from build123d import *

# Parameters (mm, degrees)
BOSS_EXTRUDE1_DEPTH = 1
SKETCH2_R           = 0.411394619
SKETCH2_R_2         = 0.305784332
SKETCH2_R_3         = 0.294014574
SKETCH2_R_4         = 0.29238352
SKETCH2_R_5         = 0.265611248
SKETCH2_R_6         = 0.339655263
SKETCH2_R_7         = 0.419941145
SKETCH2_R_8         = 0.432128273
CUT_EXTRUDE1_DEPTH  = 1
SKETCH2_5_R         = 2.453911785
BOSS_EXTRUDE2_DEPTH = 4


with BuildPart() as part:
    # Sketch1 → Boss-Extrude1 (new body)
    with BuildSketch(Plane.XY):
        with BuildLine():
            Line((-6.5, -5), (6.5, -5))
            ThreePointArc((6.5, -5), (7.207106781, -4.707106781), (7.5, -4))
            Line((7.5, -4), (7.5, 4))
            ThreePointArc((7.5, 4), (7.207106781, 4.707106781), (6.5, 5))
            Line((6.5, 5), (-6.5, 5))
            ThreePointArc((-6.5, 5), (-7.207106781, 4.707106781), (-7.5, 4))
            Line((-7.5, 4), (-7.5, -4))
            ThreePointArc((-7.5, -4), (-7.207106781, -4.707106781), (-6.5, -5))
        make_face()
    extrude(amount=BOSS_EXTRUDE1_DEPTH)

    # Sketch2 → Cut-Extrude1 (cut)
    with BuildSketch(Plane.XY.offset(1)):
        with Locations((-6.6069869, -4.252731437)):
            Circle(SKETCH2_R)
        with Locations((-2.739976181, -3.037963672)):
            Circle(SKETCH2_R_2)
        with Locations((-0.911075824, -2.990722704)):
            Circle(SKETCH2_R_3)
        with Locations((0.789599047, -2.990722704)):
            Circle(SKETCH2_R_4)
        with Locations((2.510520048, -2.990722704)):
            Circle(SKETCH2_R_5)
        with Locations((6.667725288, -4.252731437)):
            Circle(SKETCH2_R_6)
        with Locations((6.667725288, 4.061679043)):
            Circle(SKETCH2_R_7)
        with Locations((-6.6069869, 4.061679043)):
            Circle(SKETCH2_R_8)
    extrude(amount=-CUT_EXTRUDE1_DEPTH, mode=Mode.SUBTRACT)

    # Sketch2_5 → Boss-Extrude2 (add)
    with BuildSketch(Plane.XY.offset(1)):
        with Locations(Location((0, 0, 0), (0, 0, 180))):
            Circle(SKETCH2_5_R)
    extrude(amount=BOSS_EXTRUDE2_DEPTH)

    # Sketch6 → Revolve1 (revolve)
    with BuildSketch(Plane(origin=(0, 0, 0), x_dir=(0, 0, -1), z_dir=(1, 0, 0)), mode=Mode.PRIVATE) as revolve1_sk:
        Polygon((-5, 2.453911785), (-8.647016012, 2.453911785), (-8.647016012, 1.874818049), (-7.823508006, 1.280931587), (-7.823508006, 0), (-5, 0), align=None)
    revolve(revolve1_sk.sketch.rotate(Axis((0, 0, 7.823508006), (0, 0, -1)), 270), axis=Axis((0, 0, 7.823508006), (0, 0, -1)))


solid = part.part
Read the model definition and answer for the solid it produces. Units are mm, in the model's axes. A direction names the side the tool comes from. Round coordinates to 2 decimals unless told otherwise and drop trailing zeros. Loops run counter-clockwise (first coordinate to the right, second up) from the corner with the lowest first, then second, coordinate; pieces in that order, holes last. Notation, with made-up numbers: (74.5, 36.5) - (114.5, 36.5) arc R6 cw to (114.5, 42.5) - close; hole circle Ø4 at (-7, 31). An arc over 180 degrees is marked (long way). One line per question, with ' | ' between items. Start each with the question number.
Q1. Section D-D on z = 5 is taken. Give the vertices of the cut face in (x, y), plus the area to 3 significant figures.
Q2. Section B-B on x = 0 is taken. Give the vertices of the cut face in (y, z).
Q3. Find the intervals of material crossed by L1, parallel to Z at x = 2, y = -4; L2, parallel to X at y = 0, z = 2; L3, parallel to X at y = 0.25, z = 6, in increasing order.
Q4. Section A-A on y = 0 is taken. Give the vertices of the cut face in (x, z).
Q5. Section C-C on z = 0.5 is taken. Count the separate pieces of the cut face and the enclosed holes in it, plus the area to 3 significant figures.
Q6. For a pull along Y with two mould halves and no side action, classify faces 3 (the cylindrical face through (6.25, 4.08, 0.51)), 4 (the cylindrical face through (-6.195, 4.191, 0.507)), 5 (the flat face through (-2, 2, 1)), 6 (the flat face through (0.1, 5, 0.5)) as +Y half, -Y half, draft (parallel to the pull), parting line (faces both ways), or undercut.
Q7. Flat-ended cylindrical pins translate along their axes: pin 1 (2 mm diameter, centred on x = -3.5, y = -2, fed in from +Z); pin 2 (0.8 mm diameter, centred on x = -0.5, y = 0, fed in from +Z). Find the tip coordinate at first contact, or state that the pin passes through.
Q8. For faces 1 (the flat face through (-0.1, -5, 0.5)), 2 (the flat face through (0, 0, 7.824)), determine the directions among +Z, -Z, +X, -X, +Y, -Y from which every point of the face is accessible in a straight line to the end or side of a thin tool.
Established:
1) outline: circle Ø4.91 at (0, 0) | area: 18.9 mm²
2) outline: (-5, 0) - (5, 0) - (5, 1) - (2.45, 1) - (2.45, 8.65) - (1.87, 8.65) - (1.28, 7.82) - (-1.28, 7.82) - (-1.87, 8.65) - (-2.45, 8.65) - (-2.45, 1) - (-5, 1) - close
3) L1: 0 to 1 | L2: -2.45 to 2.45 | L3: -2.44 to 2.44
4) outline: (-7.5, 0) - (7.5, 0) - (7.5, 1) - (2.45, 1) - (2.45, 8.65) - (1.87, 8.65) - (1.28, 7.82) - (-1.28, 7.82) - (-1.87, 8.65) - (-2.45, 8.65) - (-2.45, 1) - (-7.5, 1) - close
5) separate pieces: 1 | enclosed holes: 8 | area: 146 mm²
6) face 3: undercut | face 4: undercut | face 5: draft | face 6: +Y half
7) pin 1: z = 1 | pin 2: z = 7.82
8) face 1: +Z, -Z, +X, -X, -Y | face 2: +Z
